```python
from build123d import *

# Parameters (mm, degrees)
SKETCH_R        = 22
PAD_DEPTH       = 7
SKETCH001_R     = 1.9
POCKET_DEPTH    = 7.001
POCKET001_DEPTH = 7.001
SKETCH003_W     = 18.5
SKETCH003_H     = 16.5
POCKET002_DEPTH = 5
POCKET003_DEPTH = 7.001
POCKET004_DEPTH = 5
CHAMFER_SIZE    = 1
CHAMFER001_SIZE = 1
CHAMFER002_SIZE = 1


with BuildPart() as part:
    # Sketch → Pad (new body)
    with BuildSketch(Plane.XY):
        Circle(SKETCH_R)
    extrude(amount=PAD_DEPTH)

    # Sketch001 → Pocket (cut, through all)
    with BuildSketch(Plane.XY.offset(7)):
        with Locations((0, 5)):
            Circle(SKETCH001_R)
    extrude(amount=-POCKET_DEPTH, mode=Mode.SUBTRACT)

    # Sketch002 → Pocket001 (cut, through all)
    with BuildSketch(Plane.XY.offset(7)):
        with BuildLine():
            ThreePointArc((21.948804, -1.5), (22, 0), (21.948804, 1.5))
            Line((21.948804, 1.5), (18.948804, 1.5))
            Line((18.948804, 1.5), (18.948804, -1.5))
            Line((18.948804, -1.5), (21.948804, -1.5))
        make_face()
    extrude(amount=-POCKET001_DEPTH, mode=Mode.SUBTRACT)

    # Sketch003 → Pocket002 (cut)
    with BuildSketch(Plane.XY.offset(7)):
        with Locations((3.293337, -8.257713)):
            Rectangle(SKETCH003_W, SKETCH003_H)
    extrude(amount=-POCKET002_DEPTH, mode=Mode.SUBTRACT)

    # Sketch004 → Pocket003 (cut, through all)
    with BuildSketch(Plane.XY.offset(7)):
        with BuildLine():
            ThreePointArc((4, 21.633308), (0, 22), (-4, 21.633308))
            Line((-4, 21.633308), (-4, 17.633308))
            Line((-4, 17.633308), (4, 17.633308))
            Line((4, 21.633308), (4, 17.633308))
        make_face()
    extrude(amount=-POCKET003_DEPTH, mode=Mode.SUBTRACT)

    # Sketch005 → Pocket004 (cut)
    with BuildSketch(Plane.XY.offset(7)):
        with BuildLine():
            ThreePointArc((0, 10.956663), (-4.212006, 9.211988), (-5.956663, 4.999975))
            Line((-5.956663, 4.999975), (-5.956663, -14.507713))
            Line((-5.956663, -14.507713), (-13.766854, -14.507713))
            ThreePointArc((16.731752, 10.956663), (-12.818201, 15.35232), (-13.766854, -14.507713))
            Line((0, 10.956663), (16.731752, 10.956663))
        make_face()
    extrude(amount=-POCKET004_DEPTH, mode=Mode.SUBTRACT)

    # Chamfer
    chamfer_edges = [part.edges().sort_by_distance(p)[0] for p in [
        (3.293337, -0.007713, 7),
    ]]
    chamfer(chamfer_edges, length=CHAMFER_SIZE)

    # Chamfer001
    chamfer001_edges = [part.edges().sort_by_distance(p)[0] for p in [
        (3.293337, -16.507713, 7),
    ]]
    chamfer(chamfer001_edges, length=CHAMFER001_SIZE)

    # Chamfer002
    chamfer002_edges = [part.edges().sort_by_distance(p)[0] for p in [
        (-5.956663, -15.507713, 7),
    ]]
    chamfer(chamfer002_edges, length=CHAMFER002_SIZE)


solid = part.part
```
Verification items for the finished model (mm, model axes). A direction names the side the tool comes from. Give positions to 0.01 mm unless a question says otherwise; leave off trailing zeros. Order: outer loops, then holes, each group sorted by start corner. A loop starts at its lowest first (then second) coordinate and runs counter-clockwise, first axis right, second up. Notation, with made-up numbers: (14, 63.5) -> (65, 63.5) arc R22 ccw to (65, 88.5) -> close; hole circle Ø7 at (36, 63). An arc over 180 degrees is marked (long way). Use a Markdown table: item, result.
1) Material ranges on probe 1 along Y at (x, z) = (0, 1.5); probe 2 along Y at (x, z) = (-7.5, 4); probe 3 along Z at (x, y) = (-0.5, 13), recorded low to high.
Results:
| item | result |
|---|---|
| probe 1 | -22 to 3.1, 6.9 to 17.63 |
| probe 2 | -20.68 to -14.51, 18.54 to 20.68 |
| probe 3 | 0 to 2 |
2) Section check B-B, the plane x = -16.5. Record the boundary of the cut face in (y, z), then the cut area to 3 significant figures.
Results:
| item | result |
|---|---|
| outline | (-14.55, 0) -> (14.55, 0) -> (14.55, 7) -> (11.3, 7) -> (11.3, 2) -> (-11.3, 2) -> (-11.3, 7) -> (-14.55, 7) -> close |
| area | 90.7 mm² |
3) Depth check by flat-ended pin: pin 1 Ø1.2 at (y, z) = (19.5, 3) entering from +X; pin 2 Ø4 at (y, z) = (-12.5, 1.5) entering from +X; pin 3 Ø3.5 at (x, z) = (21, 2) entering from +Y. Enter the tip coordinate at first touch or a pass-through.
Results:
| item | result |
|---|---|
| pin 1 | x = 11.26 |
| pin 2 | x = 19.33 |
| pin 3 | y = 10.65 |
4) Section check C-C, the plane z = 0.5. Record the boundary of the cut face in (x, y), then the cut area to 3 significant figures.
Results:
| item | result |
|---|---|
| outline | (-4, 17.63) -> (-4, 21.63) arc R22 ccw (long way) to (21.95, -1.5) -> (18.95, -1.5) -> (18.95, 1.5) -> (21.95, 1.5) arc R22 ccw to (4, 21.63) -> (4, 17.63) -> close; hole circle Ø3.8 at (0, 5) |
| area | 1,470 mm² |
5) Section check A-A, the plane z = 5. Record the boundary of the cut face in (x, y), then the cut area to 3 significant figures.
Results:
| item | result |
|---|---|
| outline | (-13.77, -14.51) arc R20 cw to (-4, 19.6) -> (-4, 21.63) arc R22 ccw (long way) to (21.95, -1.5) -> (18.95, -1.5) -> (18.95, 1.5) -> (21.95, 1.5) arc R22 ccw to (4, 21.63) -> (4, 19.6) arc R20 cw to (16.73, 10.96) -> (0, 10.96) arc R5.96 ccw to (-5.96, 5) -> (-5.96, -0.01) -> (12.54, -0.01) -> (12.54, -16.51) -> (-5.96, -16.51) -> (-5.96, -14.51) -> close; hole circle Ø3.8 at (0, 5) |
| area | 640 mm² |
6) Tool access check on faces 4 (the cylindrical face through (-0.247, 6.884, 3.549)), 5 (the flat face through (18.949, 0, 4)), 6 (the flat face through (4, 20, 3)), 7 (the flat face through (0, 0, 0)), 8 (the cylindrical face through (-19.14, 5.8, 4.54)). Record the directions out of +Z, -Z, +X, -X, +Y, -Y that give a thin tool (end or side, any length) a straight path to the whole face; none if there is none.
Results:
| item | result |
|---|---|
| face 4 | +Z, -Z |
| face 5 | +Z, -Z, +X |
| face 6 | +Z, -Z, +Y |
| face 7 | -Z, +X, -X, +Y, -Y |
| face 8 | +Z |
7) Section check D-D, the plane y = 10. Record the boundary of the cut face in (x, z).
Results:
| item | result |
|---|---|
| outline | (-19.6, 0) -> (19.6, 0) -> (19.6, 7) -> (-3.24, 7) -> (-3.24, 2) -> (-17.32, 2) -> (-17.32, 7) -> (-19.6, 7) -> close |
8) Mould release check, pull along X, two halves, no side actions. Record for faces 1 (the flat face through (-5.957, 3, 5)), 2 (the cylindrical face through (16.556, 14.488, 3.451)), 3 (the flat face through (20, 1.5, 4)): pulls with the +X half, pulls with the -X half, needs draft (parallel to the pull), parting line crosses it, or undercut.
Results:
| item | result |
|---|---|
| face 1 | undercut |
| face 2 | pulls with the +X half |
| face 3 | needs draft |
